Model file for the job. Use its own axes, mm. Coordinates: 2 decimals unless noted, no trailing zeros. Order: outer loops, then holes, each group sorted by start corner. A loop starts at its lowest first (then second) coordinate and runs counter-clockwise, first axis right, second up. Notation, with made-up numbers: M -32.5,3 L 3.5,3 A18 cw 3.5,20 Z; hole C -40,2 d9. An arc over 180 degrees is marked long. Return JSON: item names as keys, results as strings.
```python
from build123d import *

# Parameters (mm, degrees)
AUFSATZ_LINEAR_AUSTRAGEN1_DEPTH = 11.4
F_5_0_5_DURCHMESSER_BOHRUNG1_D  = 5


with BuildPart() as part:
    # Skizze1 → Aufsatz-Linear austragen1 (new body)
    with BuildSketch(Plane.XY):
        Polygon((28.7, -28.7), (28.7, 0), (28.7, 28.7), (-28.7, 28.7), (-28.7, -28.7), align=None)
    extrude(amount=AUFSATZ_LINEAR_AUSTRAGEN1_DEPTH)

    # Ø5.0 (5) Durchmesser Bohrung1 (through all)
    with Locations(Plane.XY.offset(11.4)):
        with Locations((-23.5, 23.5), (23.5, 23.5), (23.5, -23.5), (-23.5, -23.5)):
            Hole(F_5_0_5_DURCHMESSER_BOHRUNG1_D / 2)


solid = part.part
```
Item 1: Saw through at A-A (x = 23.5). Write the cut outline in (y, z).
Check result:
{"outline": "M -28.7,0 L -26,0 L -26,11.4 L -28.7,11.4 Z; M -21,0 L 21,0 L 21,11.4 L -21,11.4 Z; M 26,0 L 28.7,0 L 28.7,11.4 L 26,11.4 Z"}
Item 2: Saw through at C-C (z = 1.25). Write the cut outline in (x, y), and give its area (3 significant figures).
Check result:
{"outline": "M -28.7,-28.7 L 28.7,-28.7 L 28.7,28.7 L -28.7,28.7 Z; hole C -23.5,-23.5 d5; hole C -23.5,23.5 d5; hole C 23.5,-23.5 d5; hole C 23.5,23.5 d5", "area": "3,220 mm2"}
Item 3: Wall check: line 1 (Y direction, x = -23.5, z = 4.75); line 2 (X direction, y = -23, z = 7). Give the ranges that are in metal, low to high.
Check result:
{"line 1": "y = -28.7 to -26, -21 to 21, 26 to 28.7", "line 2": "x = -28.7 to -25.95, -21.05 to 21.05, 25.95 to 28.7"}
Item 4: Pull direction X, two halves, no side cores. Call faces 1 (the flat face through (0, 0, 0)), 2 (the flat face through (-28.7, 0, 6)), 3 (the cylindrical face through (25.34, -21.81, 5.62)): +X half, -X half, draft (parallel to the pull), parting line (faces both ways), or undercut.
Check result:
{"face 1": "draft", "face 2": "-X half", "face 3": "undercut"}
